Check sheet for the drawn part. Datum: minimum x, y, z corner. Units: mm. A direction names the side the tool comes from. Give positions to 0.01 mm unless a question says otherwise; leave off trailing zeros. Write each loop counter-clockwise with the first axis right and the second up, starting at its lowest first coordinate (ties: lowest second). Pieces come first, ordered by that corner, then holes. Notation, with made-up numbers: (69.25, 78.25) -> (75.25, 78.25) arc R29 cw to (75.25, 117.25) -> close; hole circle Ø5 at (2, -13). An arc over 180 degrees is marked (long way). Answer as CSV lines item,"result". Start each with the question number.
1) Sectioned sample at C-C on y = 38. Record the cut outline in (x, z) (1 decimal), and give its area (3 significant figures).
2) Material ranges on L1, parallel to Y at x = 101, z = 70; L2, parallel to Z at x = 82, y = 35 (1 decimal); L3, parallel to X at y = 3, z = 40 (1 decimal), recorded low to high.
3) Sectioned sample at A-A on x = 40. Record the cut outline in (y, z) (1 decimal), and give its area (3 significant figures).
4) Gauge pin test, flat ends, axial feed: pin 1 Ø5 at (x, z) = (58, 80) entering from +Y; pin 2 Ø22 at (x, y) = (79.5, 39.5) entering from +Z. Record the tip position at first contact, or that the pin passes through.
5) Sectioned sample at B-B on z = 72.5. Record the cut outline in (x, y).
6) Tool access check on the marked faces 1 and 2. Record the directions out of +Z, -Z, +X, -X, +Y, -Y that give a thin tool (end or side, any length) a straight path to the whole face; none if there is none.
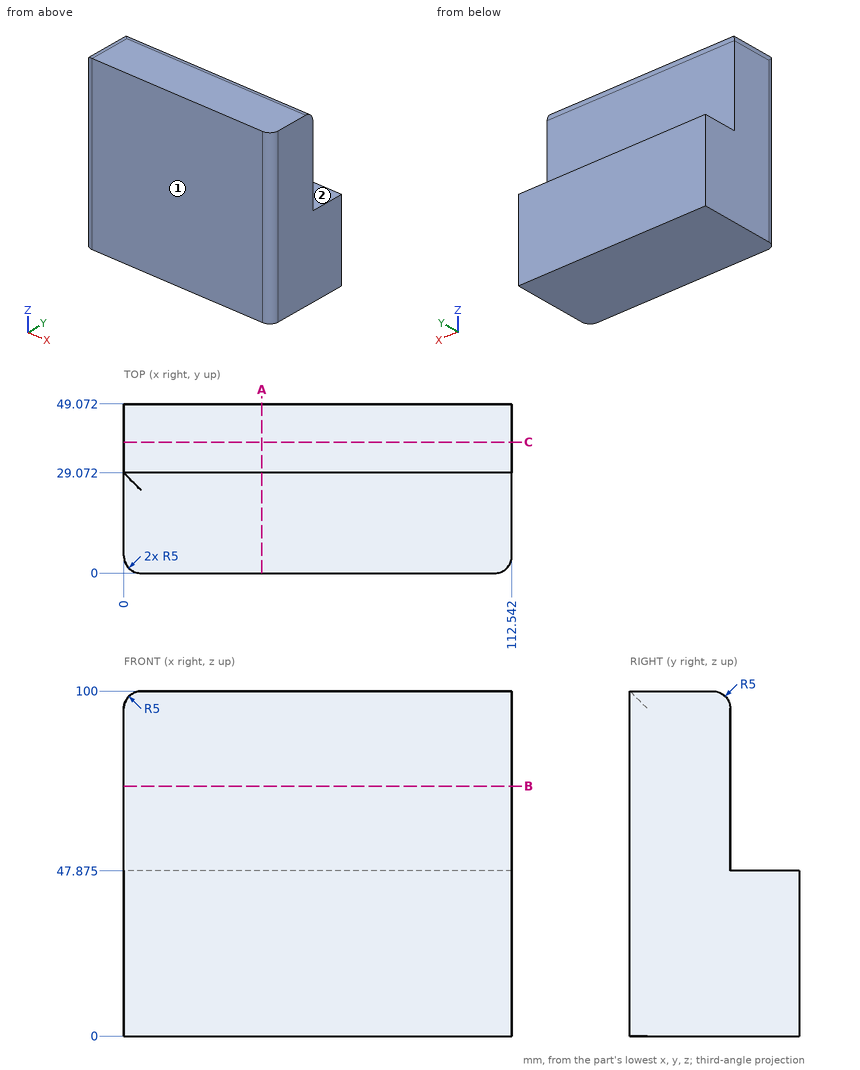
Ans:
1,outline,"(0, 0) -> (112.5, 0) -> (112.5, 47.9) -> (0, 47.9) -> close"
1,area,"5,390 mm²"
2,L1,"y = 0 to 29.07"
2,L2,"z = 0 to 47.9"
2,L3,"x = 0.4 to 112.1"
3,outline,"(0, 0) -> (49.1, 0) -> (49.1, 47.9) -> (29.1, 47.9) -> (29.1, 95) arc R5 ccw to (24.1, 100) -> (0, 100) -> close"
3,area,"3,860 mm²"
4,pin 1,"stops at y = 29.07"
4,pin 2,"stops at z = 97.32"
5,outline,"(0, 5) arc R5 ccw to (5, 0) -> (107.54, 0) arc R5 ccw to (112.54, 5) -> (112.54, 29.07) -> (0, 29.07) -> close"
6,face 1,"+Z, -Z, +X, -X, -Y"
6,face 2,"+Z, +X, -X, +Y"
